The listing builds one solid part. Answer for the finished solid, in the listing's coordinates (mm). A direction names the side the tool comes from. Give positions to 0.01 mm unless a question says otherwise; leave off trailing zeros. Loops run counter-clockwise (first coordinate to the right, second up) from the corner with the lowest first, then second, coordinate; pieces in that order, holes last. Notation, with made-up numbers: (-10.75, 49) - (8.25, 49) arc R25 ccw to (8.25, 79) - close; hole circle Ø7 at (14.5, 61). An arc over 180 degrees is marked (long way). Write each question's results on one line, items separated by ' | '.
from build123d import *

# Parameters (mm, degrees)
BOSS_EXTRUDE1_DEPTH = 13
SKETCH2_W           = 8.229441325
SKETCH2_H           = 5
CUT_EXTRUDE1_DEPTH  = 100
FILLET1_R           = 1


with BuildPart() as part:
    # Sketch1 → Boss-Extrude1 (new body)
    with BuildSketch(Plane.XY):
        Polygon((0, 0), (40, 0), (40, 43), (33, 43), (33, 3), (0, 3), align=None)
    extrude(amount=BOSS_EXTRUDE1_DEPTH)

    # Sketch2 → Cut-Extrude1 (cut)
    with BuildSketch(Plane(origin=(40, 0, 0), x_dir=(0, 0, -1), z_dir=(1, 0, 0))):
        Polygon((-3, 34), (-13, 34), (-13, 0), (-10, 0), (-10, 3), (-3, 3), align=None)
        with Locations((-7.114720663, 38.5)):
            Rectangle(SKETCH2_W, SKETCH2_H)
    extrude(amount=-CUT_EXTRUDE1_DEPTH, mode=Mode.SUBTRACT)

    # Mirror2: part across plane


with BuildPart() as part_1:
    add(part.part)
    add(part.part.mirror(Plane(origin=(0, 0, 13), x_dir=(0, 0, 1), z_dir=(1, 0, 0))))

    # Fillet1
    fillet1_edges = [part_1.edges().sort_by_distance(p)[0] for p in [
        (-40, 0, 5),
        (0, 0, 10),
        (40, 0, 5),
        (40, 1.5, 10),
        (40, 38.5, 3),
        (40, 36, 7.114720663),
        (40, 38.5, 11.229441325),
        (40, 41, 7.114720663),
        (33, 41, 7.114720663),
        (33, 3, 1.5),
        (33, 38.5, 11.229441325),
        (33, 36, 7.114720663),
        (33, 38.5, 3),
        (36.5, 3, 3),
        (0, 3, 10),
        (-36.5, 3, 3),
        (-33, 3, 1.5),
        (-33, 41, 7.114720663),
        (-33, 38.5, 11.229441325),
        (-33, 36, 7.114720663),
        (-33, 38.5, 3),
        (-40, 38.5, 3),
        (-40, 36, 7.114720663),
        (-40, 38.5, 11.229441325),
        (-40, 41, 7.114720663),
        (-36.5, 43, 0),
        (-36.5, 43, 13),
        (-36.5, 34, 13),
        (-36.5, 34, 3),
        (36.5, 34, 3),
        (36.5, 34, 13),
        (36.5, 43, 13),
        (36.5, 43, 0),
        (-40, 1.5, 10),
    ]]
    fillet(fillet1_edges, radius=FILLET1_R)


solid = part_1.part
Item 1: Find the intervals of material crossed by line 1 along Z through (x, y) = (-36, 38); line 2 along X through (y, z) = (35, 5); line 3 along Y through (x, z) = (10.5, 7.25), in increasing order. Write a range as [from, to].
Values found:
line 1: z = [0, 3], [11.23, 13] | line 2: x = [-40, -33], [33, 40] | line 3: y = [0, 3]
Item 2: Flat-ended cylindrical pins translate along their axes: P1, Ø7.5, axis at x = -37, y = 11.5, coming from the +Z side; P2, Ø4, axis at x = 20.5, y = 5.5, coming from the -Z side; P3, Ø0.5, axis at x = -19.5, y = 1.5, coming from the +Z side; P4, Ø7, axis at x = -10, z = 6.5, coming from the +Y side. Find the tip coordinate at first contact, or state that the pin passes through.
Values found:
P1: stops at z = 3 | P2: passes through | P3: stops at z = 10 | P4: stops at y = 3
Item 3: For a pull along X with two mould halves and no side action, classify faces 1 (the face through (-37, 34, 8)), 2 (the face through (40, 23, 2)), 3 (the face through (-1, 3, 4)), 4 (the face through (-33, 26.5, 2.6)) as released by +X, released by -X, zero draft, split by the parting line, or undercut.
Values found:
face 1: zero draft | face 2: released by +X | face 3: undercut | face 4: undercut
Item 4: A cutting plane is placed at C-C, the plane x = -31. Determine the outline of the cut face in (y, z).
Values found:
outline: (0, 0) - (3, 0) - (3, 9) arc R1 ccw to (2, 10) - (1, 10) arc R1 ccw to (0, 9) - close
Item 5: A cutting plane is placed at B-B, the plane z = 7. Count the separate pieces of the cut face and the enclosed holes in it, plus the area to 3 significant figures.
Values found:
separate pieces: 5 | enclosed holes: 0 | area: 294 mm²
Item 6: A cutting plane is placed at A-A, the plane y = 8.5. Determine the outline of the cut face in (x, z).
Values found:
outline: (-40, 0) - (-33, 0) - (-33, 3) - (-40, 3) - close; (33, 0) - (40, 0) - (40, 3) - (33, 3) - close
Item 7: For faces 5 (the face through (37, 36, 7)), 6 (the face through (36, 39, 13)), 7 (the face through (37, 34, 8)), 8 (the face through (33, 26.5, 2.6)), determine the directions among +Z, -Z, +X, -X, +Y, -Y from which every point of the face is accessible in a straight line to the end or side of a thin tool.
Values found:
face 5: +X, -X | face 6: +Z, +X, -X, +Y, -Y | face 7: +Z, +X, -X | face 8: +Z, -Z, +Y
